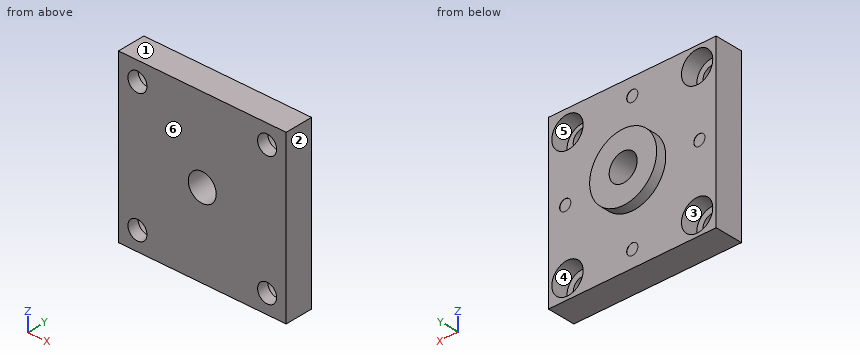
Autodesk Inventor part; units mm, degrees
ref_plane "YZ Plane" through (0, 0, 0) normal (1, 0, 0) x (0, 1, 0)
ref_plane "XZ Plane" through (0, 0, 0) normal (0, 1, 0) x (-1, 0, 0)
ref_plane "XY Plane" through (0, 0, 0) normal (0, 0, 1) x (1, 0, 0)
sketch "Sketch1" plane through (0, 0, 0) normal (0, 1, 0) x (-1, 0, 0)
  line L0 (-75, -75) -> (75, -75)
  line L1 (75, -75) -> (75, 75)
  line L2 (75, 75) -> (-75, 75)
  line L3 (-75, 75) -> (-75, -75)
  line L4 (-75, -75) -> (75, 75) construction
  line L5 (75, -75) -> (-75, 75) construction
  point P0 (0, 0)
  dimension "d0" = 150
  dimension "d1" = 150
extrude "Extrusion1" add sketch "Sketch1" along normal blind 25
sketch "Sketch2" plane through (0, 25, 0) normal (0, 1, 0) x (1, 0, 0)
  circle A0 centre (0, 0) radius 30
  dimension "d4" = 60
sketch "Sketch3" plane through (0, 25, 0) normal (0, 1, 0) x (1, 0, 0)
  line L0 (58, 58) -> (-58, 58) construction
  line L1 (-58, 58) -> (-58, -58) construction
  line L2 (-58, -58) -> (58, -58) construction
  line L3 (58, -58) -> (58, 58) construction
  line L4 (58, 58) -> (-58, -58) construction
  line L5 (-58, 58) -> (58, -58) construction
  circle A0 centre (0, 0) radius 60 construction
  point P0 (58, -56.2544)
  point P1 (0, 60)
  dimension "d7" = 120
  dimension "d5" = 116
  dimension "d6" = 116
extrude "Extrusion2" add sketch "Sketch2" along normal blind 9
hole "Hole1" at (-58, 25, -58) at (58, 25, -58) at (58, 25, 56.2544) at (-58, 25, 58) direction (0, -1, 0) diameter 28 depth 15
hole "Hole2" at (0, 25, -60) direction (0, -1, 0) diameter 10 depth 0.2
pattern_circular "Circular Pattern1" count 4 over 360 about axis through (0, 25, 0) along (0, 1, 0) of "Hole2"
sketch "Sketch5" plane through (0, 34, 0) normal (0, 1, 0) x (1, 0, 0)
  circle A0 centre (0, 0) radius 30 construction
hole "Hole5" at (0, 34, 0) direction (0, -1, 0) diameter 25 end through all
thread "Thread1"
sketch "Sketch6" plane through (58, 10, -58) normal (0, 1, 0) x (1, 0, 0)
  circle A0 centre (0, 0) radius 14 construction
  circle A1 centre (0, 0) radius 8.5
  point P0 (-58, -58)
  dimension "d50" = 17
hole "Hole6" at (58, 10, -58) direction (0, -1, 0) diameter 17 end through all
pattern_circular "Circular Pattern2" count 4 over 360 about axis through (0, 25, 0) along (0, 1, 0) of "Hole6"
properties part number "BasePlate" material "Iron, Cast"
Here's how the part is built. I have some questions about the finished solid (model axes, mm). Face numbers are marked on the shaded views. A direction names the side the tool comes from. Give positions to 0.01 mm unless a question says otherwise; leave off trailing zeros. Order: outer loops, then holes, each group sorted by start corner. A loop starts at its lowest first (then second) coordinate and runs counter-clockwise, first axis right, second up. Notation, with made-up numbers: M 7,-30.75 L 13,-30.75 A18 cw 13,-12.75 Z; hole C 87.5,-38 d10. An arc over 180 degrees is marked long. Answer as a JSON object with one key per item and string values. Group by question number.
1) On a 3-axis mill with a long thin cutter (end or side, diameter ignored), from which of +Z, -Z, +X, -X, +Y, -Y can I reach the whole of each face in a straight line? I mean the marked faces 5 and 6. Say none if no direction works.
2) We'd pull the mould along Z, two halves only. Please class the marked faces 1, 2, 3 and 4: pulls with the +Z half, pulls with the -Z half, needs draft (parallel to the pull), parting line crosses it, or undercut.
3) Suppose I cut it at D-D, the plane z = -60. Write out the boundary of the cut face in (x, y), plus the area to 3 significant figures.
4) I'm going to push flat-ended pins straight in: pin 1 Ø14 at (x, z) = (64, -53.5) entering from +Y; pin 2 Ø15.5 at (x, z) = (58, 58) entering from -Y; pin 3 Ø3 at (x, z) = (2.5, -60.5) entering from +Y; pin 4 Ø8.5 at (x, z) = (63.5, 60.5) entering from +Y. Where does each tip first touch, or does it pass through?
5) Suppose I cut it at C-C, the plane x = -53. Write out the boundary of the cut face in (y, z), plus the area to 3 significant figures.
6) Suppose I cut it at A-A, the plane y = 12.5. Write out the boundary of the cut face in (x, z).
7) Suppose I cut it at B-B, the plane z = 0. Write out the boundary of the cut face in (x, y), plus the area to 3 significant figures.
8) Please list where these lines run through material, in increasing order: L1, parallel to Z at x = 58, y = 14; L2, parallel to Z at x = 58, y = 5; L3, parallel to X at y = 7.5, z = -0.5. Write a range as [from, to].
Results found:
{
 "1": {"face 5": "+Y", "face 6": "+Z, -Z, +X, -X, -Y"},
 "2": {"face 1": "pulls with the +Z half", "face 2": "needs draft", "face 3": "undercut", "face 4": "undercut"},
 "3": {"outline": "M -75,0 L -66.26,0 L -66.26,10 L -71.86,10 L -71.86,25 L -75,25 Z; M -49.74,0 L 49.74,0 L 49.74,10 L 44.14,10 L 44.14,25 L 5,25 L 5,24.8 L -5,24.8 L -5,25 L -44.14,25 L -44.14,10 L -49.74,10 Z; M 66.26,0 L 75,0 L 75,25 L 71.86,25 L 71.86,10 L 66.26,10 Z", "area": "2,590 mm²"},
 "4": {"pin 1": "y = 25", "pin 2": "through", "pin 3": "y = 24.8", "pin 4": "y = 10"},
 "5": {"outline": "M 0,-75 L 25,-75 L 25,-71.08 L 10,-71.08 L 10,-64.87 L 0,-64.87 Z; M 0,-51.13 L 10,-51.13 L 10,-44.92 L 25,-44.92 L 25,44.92 L 10,44.92 L 10,51.13 L 0,51.13 Z; M 0,64.87 L 10,64.87 L 10,71.08 L 25,71.08 L 25,75 L 0,75 Z", "area": "2,690 mm²"},
 "6": {"outline": "M -75,-75 L 75,-75 L 75,75 L -75,75 Z; hole C -58,-58 d28; hole C -58,58 d28; hole C 0,0 d25; hole C 58,-58 d28; hole C 58,56.25 d28"},
 "7": {"outline": "M -75,0 L -12.5,0 L -12.5,34 L -30,34 L -30,25 L -55,25 L -55,24.8 L -65,24.8 L -65,25 L -75,25 Z; M 12.5,0 L 75,0 L 75,25 L 65,25 L 65,24.8 L 55,24.8 L 55,25 L 30,25 L 30,34 L 12.5,34 Z", "area": "3,440 mm²"},
 "8": {"L1": "[-75, -72], [-44, 42.25], [70.25, 75]", "L2": "[-75, -66.5], [-49.5, 49.5], [66.5, 75]", "L3": "[-75, -12.49], [12.49, 75]"}
}
